```python
from build123d import *

# Parameters (mm, degrees)
CYLINDER035_R     = 2.5
CYLINDER035_DEPTH = 10
CYLINDER034_R     = 2.5
CYLINDER034_DEPTH = 10
CYLINDER023_R     = 4.1
CYLINDER023_DEPTH = 12
CYLINDER008_R     = 4.1
CYLINDER008_DEPTH = 12
BOX001_W          = 10
BOX001_H          = 12
BOX001_DEPTH      = 83
BOX007_W          = 5
BOX007_H          = 3
BOX007_DEPTH      = 16
CYLINDER027_R     = 0.8
CYLINDER027_DEPTH = 10
CYLINDER028_R     = 0.8
CYLINDER028_DEPTH = 10
CYLINDER029_R     = 0.8
CYLINDER029_DEPTH = 10
CYLINDER_R        = 0.8
CYLINDER_DEPTH    = 10
BOX003_W          = 18
BOX003_H          = 8
BOX003_DEPTH      = 26
CYLINDER031_R     = 0.8
CYLINDER031_DEPTH = 5
CYLINDER032_R     = 0.8
CYLINDER032_DEPTH = 5
CYLINDER033_R     = 0.8
CYLINDER033_DEPTH = 5
CYLINDER030_R     = 0.8
CYLINDER030_DEPTH = 5
BOX006_W          = 4
BOX006_H          = 8
BOX006_DEPTH      = 3
BOX009_W          = 4
BOX009_H          = 8
BOX009_DEPTH      = 3
BOX005_W          = 4
BOX005_H          = 14
BOX005_DEPTH      = 50
BOX004_W          = 8
BOX004_H          = 22
BOX004_DEPTH      = 83


with BuildPart() as screwhole001:
    # Cylinder035 → Cylinder035 (new body)
    with BuildSketch(Plane(origin=(0, 6, 44), x_dir=(0, 0, -1), z_dir=(1, 0, 0))):
        Circle(CYLINDER035_R)
    extrude(amount=CYLINDER035_DEPTH)


with BuildPart() as fusion:
    # Cylinder034 → Cylinder034 (new body)
    with BuildSketch(Plane(origin=(0, 6, 64), x_dir=(0, 0, -1), z_dir=(1, 0, 0))):
        Circle(CYLINDER034_R)
    extrude(amount=CYLINDER034_DEPTH)

    # Fusion: union ScrewHole001
    add(screwhole001.part)


with BuildPart() as polea1:
    # Cylinder023 → Cylinder023 (new body)
    with BuildSketch(Plane(origin=(10, 12, 73), x_dir=(1, 0, 0), z_dir=(0, -1, 0))):
        Circle(CYLINDER023_R)
    extrude(amount=CYLINDER023_DEPTH)


with BuildPart() as polea2:
    # Cylinder008 → Cylinder008 (new body)
    with BuildSketch(Plane(origin=(10, 12, 55), x_dir=(1, 0, 0), z_dir=(0, -1, 0))):
        Circle(CYLINDER008_R)
    extrude(amount=CYLINDER008_DEPTH)


with BuildPart() as obj1:
    # Box001 → Box001 (new body)
    with BuildSketch(Plane.XY):
        with Locations((5, 6)):
            Rectangle(BOX001_W, BOX001_H)
    extrude(amount=BOX001_DEPTH)

    # Cut005: cut PoleA2
    add(polea2.part, mode=Mode.SUBTRACT)

    # Cut015: cut PoleA1
    add(polea1.part, mode=Mode.SUBTRACT)

    # Cut016: cut Fusion
    add(fusion.part, mode=Mode.SUBTRACT)


with BuildPart() as cut015:
    # Box007 → Box007 (new body)
    with BuildSketch(Plane(origin=(-8, -8, 11), x_dir=(1, 0, 0), z_dir=(0, 0, 1))):
        with Locations((2.5, 1.5)):
            Rectangle(BOX007_W, BOX007_H)
    extrude(amount=BOX007_DEPTH)


with BuildPart() as obj2:
    # Cylinder027 → Cylinder027 (new body)
    with BuildSketch(Plane(origin=(-5.35, -2, 8.85), x_dir=(1, 0, 0), z_dir=(0, -1, 0))):
        Circle(CYLINDER027_R)
    extrude(amount=CYLINDER027_DEPTH)


with BuildPart() as obj3:
    # Cylinder028 → Cylinder028 (new body)
    with BuildSketch(Plane(origin=(7.35, -2, 29.15), x_dir=(1, 0, 0), z_dir=(0, -1, 0))):
        Circle(CYLINDER028_R)
    extrude(amount=CYLINDER028_DEPTH)


with BuildPart() as obj4:
    # Cylinder029 → Cylinder029 (new body)
    with BuildSketch(Plane(origin=(-5.35, -2, 29.15), x_dir=(1, 0, 0), z_dir=(0, -1, 0))):
        Circle(CYLINDER029_R)
    extrude(amount=CYLINDER029_DEPTH)


with BuildPart() as obj5:
    # Cylinder → Cylinder (new body)
    with BuildSketch(Plane(origin=(7.35, -2, 8.85), x_dir=(1, 0, 0), z_dir=(0, -1, 0))):
        Circle(CYLINDER_R)
    extrude(amount=CYLINDER_DEPTH)

    # Fusion007: union obj2, obj3, obj4
    add(obj2.part)
    add(obj3.part)
    add(obj4.part)


with BuildPart() as obj6:
    # Box003 → Box003 (new body)
    with BuildSketch(Plane(origin=(-8, -8, 6), x_dir=(1, 0, 0), z_dir=(0, 0, 1))):
        with Locations((9, 4)):
            Rectangle(BOX003_W, BOX003_H)
    extrude(amount=BOX003_DEPTH)

    # Cut011: cut obj5
    add(obj5.part, mode=Mode.SUBTRACT)

    # Cut014: cut Cut015
    add(cut015.part, mode=Mode.SUBTRACT)


with BuildPart() as obj7:
    # Cylinder031 → Cylinder031 (new body)
    with BuildSketch(Plane(origin=(-3, 11.7, 2.5), x_dir=(0, 0, 1), z_dir=(-1, 0, 0))):
        Circle(CYLINDER031_R)
    extrude(amount=CYLINDER031_DEPTH)


with BuildPart() as obj8:
    # Cylinder032 → Cylinder032 (new body)
    with BuildSketch(Plane(origin=(-3, 0.28, 49.5), x_dir=(0, 0, 1), z_dir=(-1, 0, 0))):
        Circle(CYLINDER032_R)
    extrude(amount=CYLINDER032_DEPTH)


with BuildPart() as obj9:
    # Cylinder033 → Cylinder033 (new body)
    with BuildSketch(Plane(origin=(-3, 11.7, 49.5), x_dir=(0, 0, 1), z_dir=(-1, 0, 0))):
        Circle(CYLINDER033_R)
    extrude(amount=CYLINDER033_DEPTH)


with BuildPart() as pi_holes001:
    # Cylinder030 → Cylinder030 (new body)
    with BuildSketch(Plane(origin=(-3, 0.28, 2.5), x_dir=(0, 0, 1), z_dir=(-1, 0, 0))):
        Circle(CYLINDER030_R)
    extrude(amount=CYLINDER030_DEPTH)

    # Fusion008: union obj7, obj8, obj9
    add(obj7.part)
    add(obj8.part)
    add(obj9.part)


with BuildPart() as pi_holes001_1:
    # Fusion008 placement: moved
    add(pi_holes001.part.moved(Location((-4, 0, 31))))


with BuildPart() as headercut1:
    # Box006 → Box006 (new body)
    with BuildSketch(Plane(origin=(-12, 2, 32), x_dir=(1, 0, 0), z_dir=(0, 0, 1))):
        with Locations((2, 4)):
            Rectangle(BOX006_W, BOX006_H)
    extrude(amount=BOX006_DEPTH)


with BuildPart() as headercut:
    # Box009 → Box009 (new body)
    with BuildSketch(Plane(origin=(-12, 2, 79), x_dir=(1, 0, 0), z_dir=(0, 0, 1))):
        with Locations((2, 4)):
            Rectangle(BOX009_W, BOX009_H)
    extrude(amount=BOX009_DEPTH)

    # Fusion009: union HeaderCut1
    add(headercut1.part)


with BuildPart() as cut018:
    # Box005 → Box005 (new body)
    with BuildSketch(Plane(origin=(-12, -1, 32), x_dir=(1, 0, 0), z_dir=(0, 0, 1))):
        with Locations((2, 7)):
            Rectangle(BOX005_W, BOX005_H)
    extrude(amount=BOX005_DEPTH)

    # Cut017: cut headercut
    add(headercut.part, mode=Mode.SUBTRACT)

    # Cut018: cut pi holes001
    add(pi_holes001_1.part, mode=Mode.SUBTRACT)


with BuildPart() as obj10:
    # Box004 → Box004 (new body)
    with BuildSketch(Plane(origin=(-8, -5, 0), x_dir=(1, 0, 0), z_dir=(0, 0, 1))):
        with Locations((4, 11)):
            Rectangle(BOX004_W, BOX004_H)
    extrude(amount=BOX004_DEPTH)

    # Fusion010: union Cut018
    add(cut018.part)

    # Fusion012: union obj1, obj6
    add(obj1.part)
    add(obj6.part)


solid = obj10.part
```
Work out the finished part from the listing and answer in its coordinate system (mm). A direction names the side the tool comes from. Give positions to 0.01 mm unless a question says otherwise; leave off trailing zeros. Order: outer loops, then holes, each group sorted by start corner. A loop starts at its lowest first (then second) coordinate and runs counter-clockwise, first axis right, second up.
1. Straight lines are drawn through the part: L1, parallel to Z at x = 7.35, y = -5.4; L2, parallel to Y at x = -10.2, z = 33.5; L3, parallel to X at y = -5.55, z = 8.85. For each, find the intervals that lie inside material, in ascending order.
Result sheet:
L1: z = 6 to 8.05, 9.65 to 28.35, 29.95 to 32
L2: y = -1 to -0.52, 1.08 to 2, 10 to 10.9, 12.5 to 13
L3: x = -8 to -6.15, -4.55 to 6.55, 8.15 to 10
2. The mould has two halves that part along Z. Classify faces 1 (the flat face through (-10, 6, 79)), 2 (the flat face through (0, -3, 57)), 3 (the cylindrical face through (5.9, 6.1, 73.1)): released by +Z, released by -Z, zero draft, split by the parting line, or undercut.
Result sheet:
face 1: released by +Z
face 2: zero draft
face 3: undercut
3. Section B-B, the plane x = -10.5 is taken. Determine the outline of the cut face in (y, z).
Result sheet:
outline: (-1, 32) - (2, 32) - (2, 35) - (10, 35) - (10, 32) - (13, 32) - (13, 82) - (10, 82) - (10, 79) - (2, 79) - (2, 82) - (-1, 82) - close; hole circle Ø1.6 at (0.28, 33.5); hole circle Ø1.6 at (0.28, 80.5); hole circle Ø1.6 at (11.7, 33.5); hole circle Ø1.6 at (11.7, 80.5)
4. Each of these flat-tipped pins is pushed along its axis until it touches: P1, Ø1.8, axis at x = 6.5, z = 2, coming from the -Y side; P2, Ø2, axis at x = -10, z = 62, coming from the -Y side; P3, Ø1.5, axis at x = -9, y = 1, coming from the +Z side. Where does it stop, or does it pass through?
Result sheet:
P1: stops at y = 0
P2: stops at y = -1
P3: stops at z = 82
5. Section C-C, the plane z = 29.15 is taken. Determine the outline of the cut face in (x, y).
Result sheet:
outline: (-8, -8) - (-6.15, -8) - (-6.15, -5) - (-4.55, -5) - (-4.55, -8) - (6.55, -8) - (6.55, -2) - (8.15, -2) - (8.15, -8) - (10, -8) - (10, 12) - (0, 12) - (0, 17) - (-8, 17) - close
6. Section D-D, the plane z = 80.5 is taken. Determine the outline of the cut face in (x, y).
Result sheet:
outline: (-12, -1) - (-8, -1) - (-8, -5) - (0, -5) - (0, 0) - (10, 0) - (10, 12) - (0, 12) - (0, 17) - (-8, 17) - (-8, 13) - (-12, 13) - (-12, 12.5) - (-8, 12.5) - (-8, 10.9) - (-12, 10.9) - (-12, 10) - (-8, 10) - (-8, 2) - (-12, 2) - (-12, 1.08) - (-8, 1.08) - (-8, -0.52) - (-12, -0.52) - close
7. Section A-A, the plane x = 1 is taken. Determine the outline of the cut face in (y, z), and give its area (3 significant figures).
Result sheet:
outline: (-8, 6) - (0, 6) - (0, 0) - (12, 0) - (12, 83) - (0, 83) - (0, 32) - (-8, 32) - close; hole circle Ø5 at (6, 44); hole circle Ø5 at (6, 64)
area: 1,160 mm2
8. For faces 4 (the flat face through (0, 6, 64)), 5 (the flat face through (-4, -5, 57)), 6 (the flat face through (-5, -5, 9)), 7 (the flat face through (5, 0, 3)), determine the directions among +Z, -Z, +X, -X, +Y, -Y from which every point of the face is accessible in a straight line to the end or side of a thin tool.
Result sheet:
face 4: +X
face 5: +Z, +X, -X, -Y
face 6: -Y
face 7: -Z, +X, -Y
